Geometry check sheet. Reference: drawing and pictorial views, mm from the part's lowest x, y, z. A direction names the side the tool comes from. Coordinates: 2 decimals unless noted, no trailing zeros. Loops run counter-clockwise (first coordinate to the right, second up) from the corner with the lowest first, then second, coordinate; pieces in that order, holes last. Notation, with made-up numbers: (60, 86) -> (76, 86) arc R14 cw to (76, 105) -> close; hole circle Ø6 at (-14, 16). An arc over 180 degrees is marked (long way). Use one line per item in the form item = value.
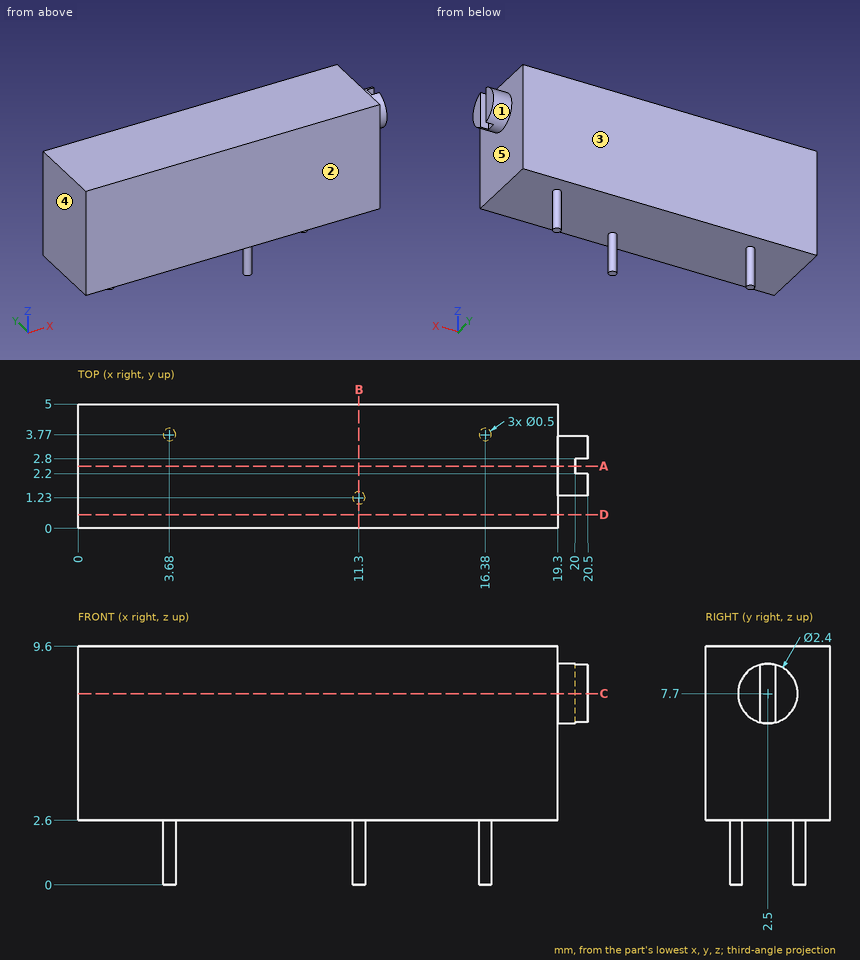
(1) Section check B-B, the plane x = 11.3. Record the boundary of the cut face in (y, z).
Established:
outline = (0, 2.6) -> (0.98, 2.6) -> (0.98, 0) -> (1.48, 0) -> (1.48, 2.6) -> (5, 2.6) -> (5, 9.6) -> (0, 9.6) -> close
(2) Mould release check, pull along X, two halves, no side actions. Record for the marked faces 3, 4 and 5: +X half, -X half, draft (parallel to the pull), parting line (faces both ways), or undercut.
Established:
face_3 = draft
face_4 = -X half
face_5 = +X half
(3) Section check C-C, the plane z = 7.7. Record the boundary of the cut face in (x, y), plus the area to 3 significant figures.
Established:
outline = (0, 0) -> (19.3, 0) -> (19.3, 1.3) -> (20.5, 1.3) -> (20.5, 2.2) -> (20, 2.2) -> (20, 2.8) -> (20.5, 2.8) -> (20.5, 3.7) -> (19.3, 3.7) -> (19.3, 5) -> (0, 5) -> close
area = 99.1 mm²
(4) Scan lines: line 1 along Z through (x, y) = (12.5, 4.7); line 2 along X through (y, z) = (2.65, 6.75); line 3 along X through (y, z) = (0.65, 3.75). Record each from-to range of solid material in increasing order.
Established:
line_1 = 2.6 to 9.6
line_2 = 0 to 20
line_3 = 0 to 19.3
(5) Go/stop test with flat-tipped pins: P1, Ø1, axis at y = 0.5, z = 8, coming from the -X side; P2, Ø1.5, axis at x = 9, y = 3, coming from the -Z side; P3, Ø2, axis at y = 3, z = 3, coming from the +X side. Record where each tip stops, or that it passes through.
Established:
P1 = 0
P2 = 2.6
P3 = 19.3
(6) Tool access check on the marked faces 1 and 2. Record the directions out of +Z, -Z, +X, -X, +Y, -Y that give a thin tool (end or side, any length) a straight path to the whole face; none if there is none.
Established:
face_1 = +X
face_2 = +Z, -Z, +X, -X, -Y
(7) Section check D-D, the plane y = 0.55. Record the boundary of the cut face in (x, z).
Established:
outline = (0, 2.6) -> (19.3, 2.6) -> (19.3, 9.6) -> (0, 9.6) -> close
(8) Section check A-A, the plane y = 2.5. Record the boundary of the cut face in (x, z), plus the area to 3 significant figures.
Established:
outline = (0, 2.6) -> (19.3, 2.6) -> (19.3, 6.5) -> (20, 6.5) -> (20, 8.9) -> (19.3, 8.9) -> (19.3, 9.6) -> (0, 9.6) -> close
area = 137 mm²
